from build123d import *

# Parameters (mm, degrees)
SKETCH_W     = 101.6
SKETCH_H     = 53.34
SKETCH_R     = 1.6
PAD_DEPTH    = 13
SKETCH001_W  = 101.91
SKETCH001_H  = 59.05
SKETCH001_R  = 1.6
PAD001_DEPTH = 22
SKETCH002_W  = 13
SKETCH002_H  = 23
PAD002_DEPTH = 17
SKETCH003_W  = 5
SKETCH003_H  = 2.5
PAD003_DEPTH = 10


with BuildPart() as part:
    # Sketch → Pad (new body)
    with BuildSketch(Plane.XY):
        with Locations((50.8, 26.67)):
            Rectangle(SKETCH_W, SKETCH_H)
        with Locations((13.97, 2.54)):
            Circle(SKETCH_R, mode=Mode.SUBTRACT)
        with Locations((15.24, 50.8)):
            Circle(SKETCH_R, mode=Mode.SUBTRACT)
        with Locations((90.17, 50.8)):
            Circle(SKETCH_R, mode=Mode.SUBTRACT)
        with Locations((96.52, 2.54)):
            Circle(SKETCH_R, mode=Mode.SUBTRACT)
        with Locations((66.04, 35.56)):
            Circle(SKETCH_R, mode=Mode.SUBTRACT)
        with Locations((66.04, 7.62)):
            Circle(SKETCH_R, mode=Mode.SUBTRACT)
    extrude(amount=-PAD_DEPTH)

    # Sketch001 (on DatumPlane) → Pad001 (join)
    with BuildSketch(Plane(origin=(0, -5.71, 0), x_dir=(1, 0, 0), z_dir=(0, 0, 1))):
        with Locations((50.955, 29.525)):
            Rectangle(SKETCH001_W, SKETCH001_H)
        with Locations((13.97, 8.25)):
            Circle(SKETCH001_R, mode=Mode.SUBTRACT)
        with Locations((15.24, 56.51)):
            Circle(SKETCH001_R, mode=Mode.SUBTRACT)
        with Locations((96.52, 8.25)):
            Circle(SKETCH001_R, mode=Mode.SUBTRACT)
    extrude(amount=PAD001_DEPTH)

    # Sketch002 (on DatumPlane) → Pad002 (join)
    with BuildSketch(Plane(origin=(0, -5.71, 0), x_dir=(1, 0, 0), z_dir=(0, 0, 1))):
        with Locations((-6.5, 11.5)):
            Rectangle(SKETCH002_W, SKETCH002_H)
    extrude(amount=PAD002_DEPTH)

    # Sketch003 (on DatumPlane) → Pad003 (join)
    with BuildSketch(Plane(origin=(0, -5.71, 0), x_dir=(1, 0, 0), z_dir=(0, 0, 1))):
        with Locations((34.5, -1.25)):
            Rectangle(SKETCH003_W, SKETCH003_H)
    extrude(amount=PAD003_DEPTH)


solid = part.part
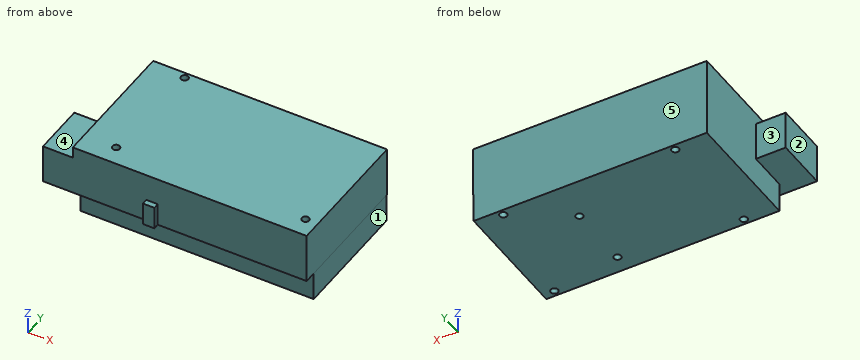
Geometry check sheet. Reference: the model listing, model coordinates, mm. Face numbers are marked on the shaded views. A direction names the side the tool comes from. Round coordinates to 2 decimals unless told otherwise and drop trailing zeros. Order: outer loops, then holes, each group sorted by start corner. A loop starts at its lowest first (then second) coordinate and runs counter-clockwise, first axis right, second up. Notation, with made-up numbers: M 43.5,-37.75 L 78.5,-37.75 A36 ccw 78.5,-1.75 Z; hole C -20.75,22 d1. An arc over 180 degrees is marked long. Answer in a Markdown table with one row per item. Add a question column.
Item 1: Set-up check for the marked faces 1, 2, 3, 4 and 5: record each of +Z, -Z, +X, -X, +Y, -Y from which the full face is reachable in a straight line by a thin tool's end or side.
Item 2: Sectioned sample at C-C, the plane x = 66.04. Enter the section's corners in (y, z).
Item 3: Sectioned sample at A-A, the plane y = 50.8. Enter the section's corners in (x, z), plus the area to 3 significant figures.
Item 4: Sectioned sample at B-B, the plane z = -8. Enter the section's corners in (x, y).
Item 5: Depth check by flat-ended pin: pin 1 Ø3.5 at (x, y) = (66.5, 35) entering from -Z; pin 2 Ø3 at (x, y) = (66.04, 7.62) entering from -Z; pin 3 Ø14.5 at (x, z) = (-8.5, 11) entering from +Y; pin 4 Ø3 at (x, y) = (96.52, 2.54) entering from +Z. Enter the tip coordinate at first touch or a pass-through.
Item 6: Sectioned sample at D-D, the plane z = 3.5. Enter the section's corners in (x, y).
Item 7: Material ranges on L1, parallel to Y at x = 66, z = -5; L2, parallel to Y at x = 90.17, z = -9.25; L3, parallel to X at y = 48.5, z = -1.5, recorded low to high. Write a range as [from, to].
Filled in:
| question | item | result |
|---|---|---|
| 1 | face 1 | -Z, +X, +Y, -Y |
| 1 | face 2 | +Z, -Z, -X, +Y, -Y |
| 1 | face 3 | +Z, -Z, -X, +Y |
| 1 | face 4 | +Z, -X, +Y, -Y |
| 1 | face 5 | +Z, -Z, +X, -X, +Y |
| 2 | outline | M -5.71,0 L 0,0 L 0,-13 L 6.02,-13 L 6.02,0 L 9.22,0 L 9.22,-13 L 33.96,-13 L 33.96,0 L 37.16,0 L 37.16,-13 L 53.34,-13 L 53.34,22 L -5.71,22 Z |
| 3 | outline | M 0,-13 L 13.64,-13 L 13.64,22 L 0,22 Z; M 16.84,-13 L 88.57,-13 L 88.57,0 L 91.77,0 L 91.77,-13 L 101.6,-13 L 101.6,0 L 101.91,0 L 101.91,22 L 16.84,22 Z |
| 3 | area | 3,410 mm² |
| 4 | outline | M 0,0 L 101.6,0 L 101.6,53.34 L 0,53.34 Z; hole C 13.97,2.54 d3.2; hole C 15.24,50.8 d3.2; hole C 66.04,7.62 d3.2; hole C 66.04,35.56 d3.2; hole C 90.17,50.8 d3.2; hole C 96.52,2.54 d3.2 |
| 5 | pin 1 | stops at z = -13 |
| 5 | pin 2 | stops at z = 0 |
| 5 | pin 3 | stops at y = 17.29 |
| 5 | pin 4 | passes through |
| 6 | outline | M -13,-5.71 L 32,-5.71 L 32,-8.21 L 37,-8.21 L 37,-5.71 L 101.91,-5.71 L 101.91,53.34 L 0,53.34 L 0,17.29 L -13,17.29 Z; hole C 13.97,2.54 d3.2; hole C 15.24,50.8 d3.2; hole C 96.52,2.54 d3.2 |
| 7 | L1 | y = [0, 6.02], [9.22, 33.96], [37.16, 53.34] |
| 7 | L2 | y = [0, 49.2], [52.4, 53.34] |
| 7 | L3 | x = [0, 101.6] |
